```python
from build123d import *

# Parameters (mm, degrees)
F0_W     = 3
F0_H     = 8
F1_DEPTH = 6


with BuildPart() as f1:
    # F0 (on Front) → F1 (new body)
    with BuildSketch(Plane.XZ):
        Polygon((0, 46), (0, 38), (-8, 38), (-8, 30), (-2, 30), (-2, 33), (0, 33), (0, 23), (6, 23), (6, 8), (0, 8), (0, 0), (10, 0), (25.4, 15.4), (25.4, 106.6), (10, 122), (0, 122), (0, 114), (-8, 114), (-8, 106), (-2, 106), (-2, 109), (0, 109), (0, 99), (6, 99), (6, 84), (0, 84), (0, 76), (-8, 76), (-8, 68), (-2, 68), (-2, 71), (0, 71), (0, 61), (6, 61), (6, 46), align=None)
        with Locations((13.5, 15)):
            Rectangle(F0_W, F0_H, mode=Mode.SUBTRACT)
        with Locations((13.5, 53)):
            Rectangle(F0_W, F0_H, mode=Mode.SUBTRACT)
        with Locations((13.5, 91)):
            Rectangle(F0_W, F0_H, mode=Mode.SUBTRACT)
    extrude(amount=F1_DEPTH)


solid = f1.part
```
Here's how the part is built. I have some questions about the finished solid (model axes, mm). A direction names the side the tool comes from. Round coordinates to 2 decimals unless told otherwise and drop trailing zeros. Order: outer loops, then holes, each group sorted by start corner. A loop starts at its lowest first (then second) coordinate and runs counter-clockwise, first axis right, second up. Notation, with made-up numbers: M -6.5,15 L 44.5,15 A14 ccw 44.5,30 Z; hole C -15,29.25 d9. An arc over 180 degrees is marked long. Use CSV: the item, a comma, the result in double quotes.
1) On a 3-axis mill with a long thin cutter (end or side, diameter ignored), from which of +Z, -Z, +X, -X, +Y, -Y can I reach the whole of each face in a straight line? I mean faces 1 (the flat face through (3, -3, 84)), 2 (the flat face through (-2, -3, 69)), 3 (the flat face through (-8, -3, 110)). Say none if no direction works.
Taken from the geometry:
face 1,"-X, +Y, -Y"
face 2,"+Y, -Y"
face 3,"+Z, -Z, -X, +Y, -Y"
2) I'm going to push flat-ended pins straight in: P1, Ø1.8, axis at y = -3.5, z = 80, coming from the -X side; P2, Ø3, axis at y = -2.5, z = 94.5, coming from the -X side; P3, Ø2, axis at x = 8.5, y = -5.5, coming from the -Z side; P4, Ø3.5, axis at x = 14, y = -4, coming from the -Z side. Where does each tip first touch, or does it pass through?
Taken from the geometry:
P1,"x = 0"
P2,"x = 6"
P3,"z = 0"
P4,"z = 2.25"
3) I want a section at C-C (y = -3.65). Count the separate pieces of the cut face and the enclosed holes in it, then the cut area to 3 significant figures.
Taken from the geometry:
separate pieces,"1"
enclosed holes,"3"
area,"2,690 mm^2"
4) I want a section at A-A (z = 93.5). List the corners of the cut face in (x, y) for me, then the cut area to 3 significant figures.
Taken from the geometry:
outline,"M 6,-6 L 12,-6 L 12,0 L 6,0 Z; M 15,-6 L 25.4,-6 L 25.4,0 L 15,0 Z"
area,"98.4 mm^2"
5) I want a section at B-B (x = 13.5). List the corners of the cut face in (y, z) for me, then the cut area to 3 significant figures.
Taken from the geometry:
outline,"M -6,3.5 L 0,3.5 L 0,11 L -6,11 Z; M -6,19 L 0,19 L 0,49 L -6,49 Z; M -6,57 L 0,57 L 0,87 L -6,87 Z; M -6,95 L 0,95 L 0,118.5 L -6,118.5 Z"
area,"546 mm^2"
6) I need wall thicknesses on line 1 along Z through (x, y) = (1, -2.55); line 2 along Z through (x, y) = (-6, -5.7); line 3 along Z through (x, y) = (14, -5.2). Which ranges of each line are inside material? Lowest first, please. Write a range as [from, to].
Taken from the geometry:
line 1,"[0, 8], [23, 46], [61, 84], [99, 122]"
line 2,"[30, 38], [68, 76], [106, 114]"
line 3,"[4, 11], [19, 49], [57, 87], [95, 118]"
7) If we mould it in two halves opening along X, with no side actions, what happens to faces 4 (the flat face through (-4, -3, 114)), 5 (the flat face through (-2, -3, 31)), 6 (the flat face through (25.4, -3, 60))? For each: pulls with the +X half, pulls with the -X half, needs draft (parallel to the pull), parting line crosses it, or undercut.
Taken from the geometry:
face 4,"needs draft"
face 5,"undercut"
face 6,"pulls with the +X half"
8) I want a section at D-D (x = 4.5). List the corners of the cut face in (y, z) for me, then the cut area to 3 significant figures.
Taken from the geometry:
outline,"M -6,0 L 0,0 L 0,8 L -6,8 Z; M -6,23 L 0,23 L 0,46 L -6,46 Z; M -6,61 L 0,61 L 0,84 L -6,84 Z; M -6,99 L 0,99 L 0,122 L -6,122 Z"
area,"462 mm^2"
